Could you check a few things on this model? Use its own coordinates, in mm. A direction names the side the tool comes from. Coordinates: 2 decimals unless noted, no trailing zeros. Order: outer loops, then holes, each group sorted by start corner. A loop starts at its lowest first (then second) coordinate and runs counter-clockwise, first axis right, second up. Notation, with made-up numbers: (-16.75, 17) -> (27.25, 17) arc R25 cw to (27.25, 29) -> close; hole circle Ø5 at (40.25, 15.25). An arc over 180 degrees is marked (long way). Return JSON: item names as keys, results as strings. Group by question number.
from build123d import *

# Parameters (mm, degrees)
F3_DEPTH = 50
F4_R     = 5


# Not quite as in the source:
# - a pattern or mirror of a feature is missing from the dataset's text; its kind, count and spacing are read off the source's solid


with BuildPart() as f1:
    # F0 (on Right) → F1 (revolve)
    with BuildSketch(Plane.YZ):
        Polygon((-55, -150), (-55, -200), (-50, -200), (-50, -300), (0, -300), (0, 300), (-50, 300), (-50, 200), (-55, 200), (-55, 150), (-50, 150), (-50, 50), (-60, 50), (-60, -50), (-50, -50), (-50, -150), align=None)
    revolve(axis=Axis((0, 0, 0), (0, 0, -1)))

    # F2 (on face) → F3 (cut)
    with BuildSketch(Plane(origin=(0, 0, -300), x_dir=(1, 0, 0), z_dir=(0, 0, -1))):
        with BuildLine():
            Line((-8.3391469531, -41.2996818255), (-8.3391469531, -49.2996818255))
            ThreePointArc((-8.3391469531, -49.2996818255), (-0.8487525257, -49.9927956725), (6.6608530469, -49.5543442766))
            Line((6.6608530469, -49.5543442766), (6.6608530469, -41.2996818255))
            Line((6.6608530469, -41.2996818255), (-8.3391469531, -41.2996818255))
        make_face()
    f3 = extrude(amount=-F3_DEPTH, mode=Mode.SUBTRACT)

    # F3_copies: F3 across plane
    add(f3.mirror(Plane.XY), mode=Mode.SUBTRACT)

    # F4
    f4_edges = [f1.edges().sort_by_distance(p)[0] for p in [
        (6.660853, 45.427013, -250),
        (-8.339147, 45.299682, -250),
        (6.660853, 45.427013, 250),
        (-8.339147, 45.299682, 250),
    ]]
    fillet(f4_edges, radius=F4_R)


solid = f1.part
Q1. I want a section at B-B on x = -19. Please give me the cut outline in (y, z), and give its area (3 significant figures).
Q2. I want a section at A-A on y = 0. Please give me the cut outline in (x, z).
Q3. I need wall thicknesses on line 1 along Z through (x, y) = (45, 27); line 2 along Z through (x, y) = (14, -54); line 3 along Y through (x, z) = (3, 31). Which ranges of each line are inside material? Lowest first, please. Write a range as from..to.
Q4. I'm going to push flat-ended pins straight in: pin 1 Ø2.5 at (y, z) = (45, 288.5) entering from +X; pin 2 Ø2.5 at (y, z) = (47.5, 266.5) entering from -X; pin 3 Ø3 at (x, z) = (-10.5, 204.5) entering from +Y. Where does each tip first touch, or does it pass through?
Q5. I want a section at D-D on z = -41.5. Please give me the cut outline in (x, y).
Q6. I want a section at C-C on z = 189.5. Please give me the cut outline in (x, y), and give its area (3 significant figures).
Q7. We'd pull the mould along Z, two halves only. Please class faces 4 (the flat face through (-45, 23, -50)), 5 (the flat face through (-1, 41.3, -275)), 6 (the flat face through (49, -12, -200)), 7 (the flat face through (-45, -23, 50)): pulls with the +Z half, pulls with the -Z half, needs draft (parallel to the pull), parting line crosses it, or undercut.
Q8. On a 3-axis mill with a long thin cutter (end or side, diameter ignored), from which of +Z, -Z, +X, -X, +Y, -Y can I reach the whole of each face in a straight line? I mean faces 1 (the cylindrical face through (-15.02, -47.69, 249.3)), 2 (the cylindrical face through (-15.02, -47.69, -250.7)), 3 (the cylindrical face through (-15.02, -47.69, 99.3)). Say none if no direction works.
Response values:
{
 "1": {"outline": "(-56.91, -50) -> (-46.25, -50) -> (-46.25, -150) -> (-51.61, -150) -> (-51.61, -200) -> (-46.25, -200) -> (-46.25, -300) -> (46.25, -300) -> (46.25, -200) -> (51.61, -200) -> (51.61, -150) -> (46.25, -150) -> (46.25, -50) -> (56.91, -50) -> (56.91, 50) -> (46.25, 50) -> (46.25, 150) -> (51.61, 150) -> (51.61, 200) -> (46.25, 200) -> (46.25, 300) -> (-46.25, 300) -> (-46.25, 200) -> (-51.61, 200) -> (-51.61, 150) -> (-46.25, 150) -> (-46.25, 50) -> (-56.91, 50) -> close", "area": "58,700 mm²"},
 "2": {"outline": "(-60, -50) -> (-50, -50) -> (-50, -150) -> (-55, -150) -> (-55, -200) -> (-50, -200) -> (-50, -300) -> (50, -300) -> (50, -200) -> (55, -200) -> (55, -150) -> (50, -150) -> (50, -50) -> (60, -50) -> (60, 50) -> (50, 50) -> (50, 150) -> (55, 150) -> (55, 200) -> (50, 200) -> (50, 300) -> (-50, 300) -> (-50, 200) -> (-55, 200) -> (-55, 150) -> (-50, 150) -> (-50, 50) -> (-60, 50) -> close"},
 "3": {"line 1": "z = -200..-150, -50..50, 150..200", "line 2": "z = -50..50", "line 3": "y = -59.92..59.92"},
 "4": {"pin 1": "stops at x = 24.21", "pin 2": "stops at x = -19", "pin 3": "stops at y = 49.18"},
 "5": {"outline": "circle Ø120 at (0, 0)"},
 "6": {"outline": "circle Ø110 at (0, 0)", "area": "9,500 mm²"},
 "7": {"face 4": "undercut", "face 5": "needs draft", "face 6": "pulls with the -Z half", "face 7": "undercut"},
 "8": {"face 1": "+Z", "face 2": "-Z", "face 3": "none"}
}
